from build123d import *

# Parameters (mm, degrees)
CYLINDER001_R     = 1.5
CYLINDER001_DEPTH = 6
CYLINDER002_R     = 1.5
CYLINDER002_DEPTH = 6
CYLINDER_R        = 1.5
CYLINDER_DEPTH    = 6
CYLINDER003_R     = 1.5
CYLINDER003_DEPTH = 6
BOX001_W          = 50
BOX001_H          = 90
BOX001_DEPTH      = 15
CHAMFER_SIZE      = 3
BOX_W             = 58
BOX_H             = 98
BOX_DEPTH         = 19
FILLET_R          = 3


with BuildPart() as cylinder001:
    # Cylinder001 → Cylinder001 (new body)
    with BuildSketch(Plane(origin=(55.5, 2.5, 19), x_dir=(1, 0, 0), z_dir=(0, 0, 1))):
        Circle(CYLINDER001_R)
    extrude(amount=CYLINDER001_DEPTH)


with BuildPart() as cylinder002:
    # Cylinder002 → Cylinder002 (new body)
    with BuildSketch(Plane(origin=(2.5, 95.5, 19), x_dir=(1, 0, 0), z_dir=(0, 0, 1))):
        Circle(CYLINDER002_R)
    extrude(amount=CYLINDER002_DEPTH)


with BuildPart() as cylinder:
    # Cylinder → Cylinder (new body)
    with BuildSketch(Plane(origin=(2.5, 2.5, 19), x_dir=(1, 0, 0), z_dir=(0, 0, 1))):
        Circle(CYLINDER_R)
    extrude(amount=CYLINDER_DEPTH)


with BuildPart() as cylinder003:
    # Cylinder003 → Cylinder003 (new body)
    with BuildSketch(Plane(origin=(55.5, 95.5, 19), x_dir=(1, 0, 0), z_dir=(0, 0, 1))):
        Circle(CYLINDER003_R)
    extrude(amount=CYLINDER003_DEPTH)


with BuildPart() as chamfer_body:
    # Box001 → Box001 (new body)
    with BuildSketch(Plane(origin=(4, 4, 4), x_dir=(1, 0, 0), z_dir=(0, 0, 1))):
        with Locations((25, 45)):
            Rectangle(BOX001_W, BOX001_H)
    extrude(amount=BOX001_DEPTH)

    # Chamfer
    chamfer_edges = [chamfer_body.edges().sort_by_distance(p)[0] for p in [
        (4, 49, 4),
        (54, 49, 4),
        (29, 4, 4),
        (29, 94, 4),
    ]]
    chamfer(chamfer_edges, length=CHAMFER_SIZE)


with BuildPart() as fusion:
    # Box → Box (new body)
    with BuildSketch(Plane.XY):
        with Locations((29, 49)):
            Rectangle(BOX_W, BOX_H)
    extrude(amount=BOX_DEPTH)

    # Cut: cut Chamfer body
    add(chamfer_body.part, mode=Mode.SUBTRACT)

    # Fillet
    fillet_edges = [fusion.edges().sort_by_distance(p)[0] for p in [
        (0, 49, 0),
        (29, 0, 0),
        (58, 49, 0),
    ]]
    fillet(fillet_edges, radius=FILLET_R)

    # Fusion: union Cylinder001, Cylinder002, Cylinder, Cylinder003
    add(cylinder001.part)
    add(cylinder002.part)
    add(cylinder.part)
    add(cylinder003.part)


solid = fusion.part
Geometry check sheet. Reference: the model listing, model coordinates, mm. A direction names the side the tool comes from. Coordinates: 2 decimals unless noted, no trailing zeros. Loops run counter-clockwise (first coordinate to the right, second up) from the corner with the lowest first, then second, coordinate; pieces in that order, holes last. Notation, with made-up numbers: (-15, 4) - (13, 4) arc R25 cw to (13, 16) - close; hole circle Ø1 at (-3.75, 67). An arc over 180 degrees is marked (long way). Use one line per item in the form item = value. Start each with the question number.
Item 1: Gauge pin test, flat ends, axial feed: pin 1 (17.5 mm diameter, centred on x = 21, y = 63, fed in from +Z); pin 2 (6 mm diameter, centred on x = 51.5, y = 25, fed in from +Z). Record the tip position at first contact, or that the pin passes through.
Item 2: Section check D-D, the plane y = 28. Enter the section's corners in (x, z), and give its area (3 significant figures).
Item 3: Section check C-C, the plane y = 95.5. Enter the section's corners in (x, z).
Item 4: Section check A-A, the plane z = 13.5. Enter the section's corners in (x, y).
Item 5: Section check B-B, the plane x = 14. Enter the section's corners in (y, z), and give its area (3 significant figures).
Item 6: Mould release check, pull along X, two halves, no side actions. Record for faces 1 (the face through (58, 48, 11)), 2 (the face through (0, 48, 11)), 3 (the face through (54, 48, 13)), 4 (the face through (55, 96, 25)): +X half, -X half, draft (parallel to the pull), parting line (faces both ways), or undercut.
Item 7: Thickness scan on probe 1 along Y at (x, z) = (32, 9.5); probe 2 along X at (y, z) = (90.5, 9.5); probe 3 along Z at (x, y) = (17.5, 32). Record the ranges inside material, lowest first.
Item 8: Tool access check on faces 5 (the face through (56.93, 2.95, 21.96)), 6 (the face through (2, 3, 25)). Record the directions out of +Z, -Z, +X, -X, +Y, -Y that give a thin tool (end or side, any length) a straight path to the whole face; none if there is none.
Computed:
q1.pin_1 = 4
q1.pin_2 = 19
q2.outline = (0, 3) arc R3 ccw to (3, 0) - (55, 0) arc R3 ccw to (58, 3) - (58, 19) - (54, 19) - (54, 7) - (51, 4) - (7, 4) - (4, 7) - (4, 19) - (0, 19) - close
q2.area = 357 mm2
q3.outline = (0, 3) arc R3 ccw to (3, 0) - (55, 0) arc R3 ccw to (58, 3) - (58, 19) - (57, 19) - (57, 25) - (54, 25) - (54, 19) - (4, 19) - (4, 25) - (1, 25) - (1, 19) - (0, 19) - close
q4.outline = (0, 0) - (58, 0) - (58, 98) - (0, 98) - close; hole (4, 4) - (54, 4) - (54, 94) - (4, 94) - close
q5.outline = (0, 3) arc R3 ccw to (3, 0) - (98, 0) - (98, 19) - (94, 19) - (94, 7) - (91, 4) - (7, 4) - (4, 7) - (4, 19) - (0, 19) - close
q5.area = 519 mm2
q6.face_1 = +X half
q6.face_2 = -X half
q6.face_3 = undercut
q6.face_4 = draft
q7.probe_1 = 0 to 4, 94 to 98
q7.probe_2 = 0 to 4, 54 to 58
q7.probe_3 = 0 to 4
q8.face_5 = +Z
q8.face_6 = +Z, +X, -X, +Y, -Y
